Answer from the drawing. Dimensions are ordinates in mm from the lowest x, y and z of the part. A direction names the side the tool comes from. Coordinates: 2 decimals unless noted, no trailing zeros. Write each loop counter-clockwise with the first axis right and the second up, starting at its lowest first coordinate (ties: lowest second). Pieces come first, ordered by that corner, then holes. Notation, with made-up numbers: (55, -23) - (79, -23) arc R17 ccw to (79, -7) - close; hole circle Ø5 at (-32, 48). An arc over 180 degrees is marked (long way). Use one line per item in the form item = value. Start each with the question number.
Item 1: Consider probe 1 along Y at (x, z) = (35.5, 0.3); probe 2 along Z at (x, y) = (29, 41); probe 3 along Z at (x, y) = (65, 41). Determine where each line is inside the solid, lowest interval first.
Item 2: A cutting plane is placed at C-C (y = 46.5). Write down the section's boundary in (x, z).
Item 3: Determine the mould class of the marked faces 1, 2 and 3 for opening direction Y: released by +Y, released by -Y, zero draft, split by the parting line, or undercut.
Item 4: A cutting plane is placed at A-A (y = 35.5). Write down the section's boundary in (x, z), then the cut area to 3 significant figures.
Item 5: Given pin 1 (10 mm diameter, centred on x = 23, y = 49.5, fed in from +Z); pin 2 (1 mm diameter, centred on x = 16, y = 53.5, fed in from -Z); pin 3 (5 mm diameter, centred on y = 46.5, z = 1, fed in from -X), each flat-ended and moving along its own axis, determine where each tip first touches the part or whether it passes through.
Item 6: A cutting plane is placed at D-D (z = 4.75). Write down the section's boundary in (x, y).
Item 7: For the marked faces 4 and 5, determine the directions among +Z, -Z, +X, -X, +Y, -Y from which every point of the face is accessible in a straight line to the end or side of a thin tool.
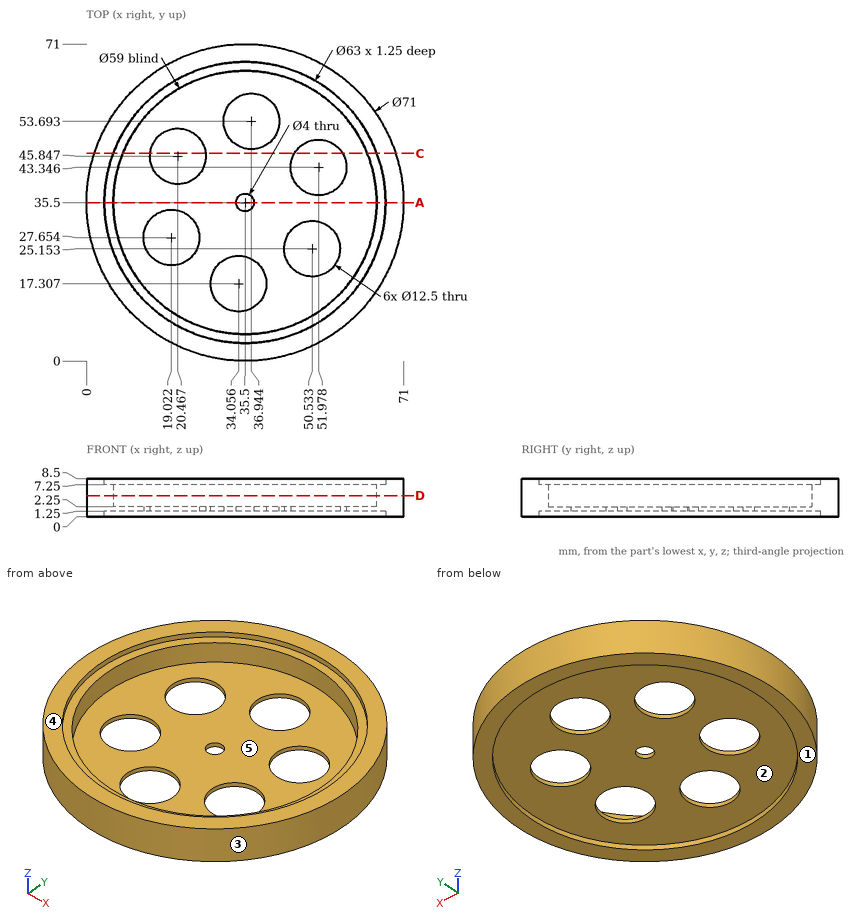
Answer:
q1.probe_1 = 0 to 4, 67 to 71
q1.probe_2 = 1.25 to 2.25
q1.probe_3 = 1.25 to 7.25
q2.outline = (1.75, 0) - (5.98, 0) - (5.98, 1.25) - (14.25, 1.25) - (14.25, 2.25) - (8.13, 2.25) - (8.13, 7.25) - (5.98, 7.25) - (5.98, 8.5) - (1.75, 8.5) - close; (26.68, 1.25) - (46.58, 1.25) - (46.58, 2.25) - (26.68, 2.25) - close; (57.37, 1.25) - (65.02, 1.25) - (65.02, 0) - (69.25, 0) - (69.25, 8.5) - (65.02, 8.5) - (65.02, 7.25) - (62.87, 7.25) - (62.87, 2.25) - (57.37, 2.25) - close
q3.face_1 = zero draft
q3.face_2 = undercut
q3.face_3 = split by the parting line
q4.outline = (0, 0) - (4, 0) - (4, 1.25) - (33.5, 1.25) - (33.5, 2.25) - (6, 2.25) - (6, 7.25) - (4, 7.25) - (4, 8.5) - (0, 8.5) - close; (37.5, 1.25) - (67, 1.25) - (67, 0) - (71, 0) - (71, 8.5) - (67, 8.5) - (67, 7.25) - (65, 7.25) - (65, 2.25) - (37.5, 2.25) - close
q4.area = 147 mm²
q5.pin_1 = 2.25
q5.pin_2 = 1.25
q5.pin_3 = 1.03
q6.outline = circle Ø71 at (35.5, 35.5); hole circle Ø59 at (35.5, 35.5)
q7.face_4 = +Z, +X, -X, +Y, -Y
q7.face_5 = +Z
